```python
from build123d import *

# Parameters (mm, degrees)
SKETCH2_W           = 156.4
SKETCH2_H           = 69
BOSS_EXTRUDE1_DEPTH = 3.175
SKETCH4_R           = 1.6
CUT_EXTRUDE1_DEPTH  = 86.531109107
SKETCH6_R           = 1.5875
CUT_EXTRUDE2_DEPTH  = 86.531109107
SKETCH7_R           = 1.5
CUT_EXTRUDE3_DEPTH  = 86.531109107
SKETCH8_W           = 146.78
SKETCH8_H           = 24.86
CUT_EXTRUDE4_DEPTH  = 86.531109107
SKETCH10_R          = 1.6
CUT_EXTRUDE6_DEPTH  = 86.531109107
SKETCH11_W          = 148.78
SKETCH11_H          = 26.86
CUT_EXTRUDE7_DEPTH  = 86.531109107
SKETCH12_W          = 20
SKETCH12_H          = 10
CUT_EXTRUDE8_DEPTH  = 86.531109107
FILLET1_R           = 5


with BuildPart() as part:
    # Sketch2 → Boss-Extrude1 (new body)
    with BuildSketch(Plane(origin=(0, 0, 0), x_dir=(1, 0, 0), z_dir=(0, 1, 0))):
        Rectangle(SKETCH2_W, SKETCH2_H)
    extrude(amount=BOSS_EXTRUDE1_DEPTH)

    # Sketch4 → Cut-Extrude1 (cut, through all)
    with BuildSketch(Plane(origin=(0, 3.175, 0), x_dir=(1, 0, 0), z_dir=(0, 1, 0))):
        with Locations(Location((71.2, -23.5, 0), (0, 0, 270))):
            Circle(SKETCH4_R)
        with Locations(Location((71.2, 23.5, 0), (0, 0, 90))):
            Circle(SKETCH4_R)
        with Locations(Location((-71.2, 23.5, 0), (0, 0, 270))):
            Circle(SKETCH4_R)
        with Locations(Location((-71.2, -23.5, 0), (0, 0, 90))):
            Circle(SKETCH4_R)
    extrude(amount=-CUT_EXTRUDE1_DEPTH, mode=Mode.SUBTRACT)

    # Sketch6 → Cut-Extrude2 (cut, through all)
    with BuildSketch(Plane.XZ):
        with Locations(Location((49.09, -29.25, 0), (0, 0, 270))):
            Circle(SKETCH6_R)
        with Locations(Location((21.15, -29.25, 0), (0, 0, 270))):
            Circle(SKETCH6_R)
        with Locations(Location((64.33, 21.55, 0), (0, 0, 270))):
            Circle(SKETCH6_R)
        with Locations(Location((16.07, 22.82, 0), (0, 0, 270))):
            Circle(SKETCH6_R)
    extrude(amount=-CUT_EXTRUDE2_DEPTH, mode=Mode.SUBTRACT)

    # Sketch7 → Cut-Extrude3 (cut, through all)
    with BuildSketch(Plane(origin=(0, 0, 0), x_dir=(-1, 0, 0), z_dir=(0, -1, 0))):
        with Locations(Location((63.2, -20.32, 0), (0, 0, 90))):
            Circle(SKETCH7_R)
        with Locations(Location((63.2, 20.32, 0), (0, 0, 270))):
            Circle(SKETCH7_R)
    extrude(amount=-CUT_EXTRUDE3_DEPTH, mode=Mode.SUBTRACT)

    # Sketch8 → Cut-Extrude4 (cut, through all)
    with BuildSketch(Plane.XZ):
        Rectangle(SKETCH8_W, SKETCH8_H)
    extrude(amount=-CUT_EXTRUDE4_DEPTH, mode=Mode.SUBTRACT)

    # Sketch10 → Cut-Extrude6 (cut, through all)
    with BuildSketch(Plane(origin=(0, 3.175, 0), x_dir=(1, 0, 0), z_dir=(0, 1, 0))):
        with Locations(Location((-7.5, -25, 0), (0, 0, 270))):
            Circle(SKETCH10_R)
        with Locations(Location((7.5, -25, 0), (0, 0, 270))):
            Circle(SKETCH10_R)
        with Locations(Location((7.5, 25, 0), (0, 0, 270))):
            Circle(SKETCH10_R)
        with Locations(Location((-7.5, 25, 0), (0, 0, 270))):
            Circle(SKETCH10_R)
    extrude(amount=-CUT_EXTRUDE6_DEPTH, mode=Mode.SUBTRACT)

    # Sketch11 → Cut-Extrude7 (cut, through all)
    with BuildSketch(Plane.XZ):
        Rectangle(SKETCH11_W, SKETCH11_H)
    extrude(amount=-CUT_EXTRUDE7_DEPTH, mode=Mode.SUBTRACT)

    # Sketch12 → Cut-Extrude8 (cut, through all)
    with BuildSketch(Plane.XZ):
        with Locations((-28.2, -23.965)):
            Rectangle(SKETCH12_W, SKETCH12_H)
        with Locations((-28.2, 23.965)):
            Rectangle(SKETCH12_W, SKETCH12_H)
    extrude(amount=-CUT_EXTRUDE8_DEPTH, mode=Mode.SUBTRACT)

    # Fillet1
    fillet1_edges = [part.edges().sort_by_distance(p)[0] for p in [
        (78.2, 1.5875, 34.5),
        (-78.2, 1.5875, 34.5),
        (-78.2, 1.5875, -34.5),
        (78.2, 1.5875, -34.5),
    ]]
    fillet(fillet1_edges, radius=FILLET1_R)


solid = part.part
```
Could you check a few things on this model? Use its own coordinates, in mm. A direction names the side the tool comes from. Round coordinates to 2 decimals unless told otherwise and drop trailing zeros. Order: outer loops, then holes, each group sorted by start corner. A loop starts at its lowest first (then second) coordinate and runs counter-clockwise, first axis right, second up. Notation, with made-up numbers: M 25,79 L 48,79 A19 cw 48,91 Z; hole C -18,42.25 d8. An arc over 180 degrees is marked long. One line per question, with ' | ' between items. Start each with the question number.
(1) For faces 1 (the face through (-28, 2, 18.965)), 2 (the face through (-1, 2, -34.5)), which set-ups out of +Z, -Z, +X, -X, +Y, -Y let a thin tool reach every point of the face, with its end or its side?
(2) Suppose I cut it at A-A on x = -59. List the corners of the cut face in (y, z) for me (3 decimals), then the cut area to 3 significant figures.
(3) Suppose I cut it at B-B on z = -5.5. List the corners of the cut face in (x, y) for me (3 decimals).
(4) Please list where these lines run through material, in increasing order: line 1 along Z through (x, y) = (-37.5, 1.8) (3 decimals); line 2 along X through (y, z) = (1.9, -29.25); line 3 along Z through (x, y) = (71.2, 2.1).
(5) For P1, Ø2.5, axis at x = -63.2, z = -20.32, coming from the +Y side, with a flat end and sliding along its axis, tell me the tip position at first contact or that it passes through.
(6) Suppose I cut it at C-C on y = 2.6. Count the separate pieces of the cut face and the enclosed holes in it, then the cut area to 3 significant figures.
(7) Thinking about a two-plate mould opening in Z: for faces 3 (the face through (78.2, 2, 0)), 4 (the face through (76.7, 1.61, 33.07)), 5 (the face through (74.39, 2, 0)), which applies, +Z half, -Z half, draft (parallel to the pull), parting line (faces both ways), or undercut?
Geometry results:
1) face 1: +Y, -Y | face 2: -Z, +X, -X, +Y, -Y
2) outline: M 0,-34.5 L 3.175,-34.5 L 3.175,-13.43 L 0,-13.43 Z; M 0,13.43 L 3.175,13.43 L 3.175,34.5 L 0,34.5 Z | area: 134 mm²
3) outline: M -78.2,0 L -74.39,0 L -74.39,3.175 L -78.2,3.175 Z; M 74.39,0 L 78.2,0 L 78.2,3.175 L 74.39,3.175 Z
4) line 1: -34.5 to -28.965, -18.965 to -13.43, 13.43 to 18.965, 28.965 to 34.5 | line 2: -78.2 to 19.56, 22.74 to 47.5, 50.68 to 78.2 | line 3: -34.5 to -25.1, -21.9 to -13.43, 13.43 to 21.9, 25.1 to 34.5
5) P1: through
6) separate pieces: 1 | enclosed holes: 17 | area: 6,260 mm²
7) face 3: draft | face 4: +Z half | face 5: undercut
